from build123d import *

# Parameters (mm, degrees)
F0_W     = 90
F0_H     = 11
F0_R     = 2.15
F0_R_2   = 2.25
F1_DEPTH = 7
F2_W     = 5
F2_H     = 5
F3_DEPTH = 8
F4_R     = 5
F5_R     = 2.99999


# Not quite as in the source:
# - a fillet or chamfer is up to 0.001 mm smaller than in the source, because OpenCascade refuses the exact size


with BuildPart() as f1:
    # F0 (on Top) → F1 (new body)
    with BuildSketch(Plane.XY):
        Rectangle(F0_W, F0_H)
        with Locations((-40, 0)):
            Circle(F0_R, mode=Mode.SUBTRACT)
        Circle(F0_R_2, mode=Mode.SUBTRACT)
        with Locations((40, 0)):
            Circle(F0_R, mode=Mode.SUBTRACT)
        Circle(F0_R_2)
    extrude(amount=F1_DEPTH)

    # F2 (on face) → F3 (join)
    with BuildSketch(Plane.XY.offset(7)):
        Rectangle(F2_W, F2_H)
    extrude(amount=F3_DEPTH)

    # F4
    f4_edges = [f1.edges().sort_by_distance(p)[0] for p in [
        (45, -5.5, 3.5),
        (45, 5.5, 3.5),
        (-45, -5.5, 3.5),
        (-45, 5.5, 3.5),
    ]]
    fillet(f4_edges, radius=F4_R)

    # F5 (radius 3 in the source; OpenCascade refuses exactly that, so slightly less here)
    f5_edges = [f1.edges().sort_by_distance(p)[0] for p in [
        (0, -5.5, 7),
    ]]
    fillet(f5_edges, radius=F5_R)


solid = f1.part
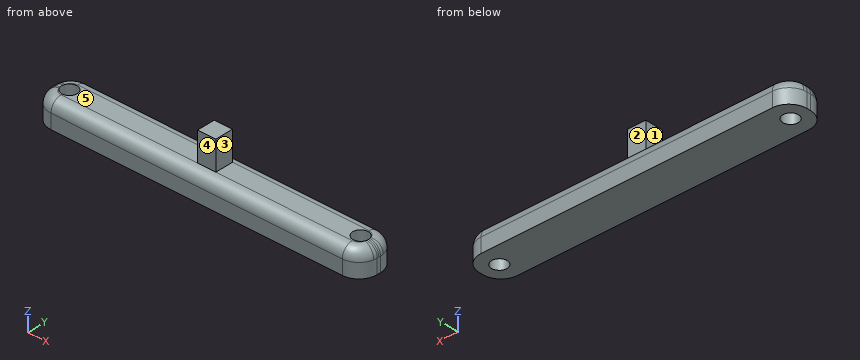
Design review of the part built by this model. Coordinates are the model's own, in mm. Face numbers are marked on the shaded views. A direction names the side the tool comes from. Coordinates: 2 decimals unless noted, no trailing zeros. Order: outer loops, then holes, each group sorted by start corner. A loop starts at its lowest first (then second) coordinate and runs counter-clockwise, first axis right, second up. Notation, with made-up numbers: (73.5, 78) -> (112.5, 78) arc R14 cw to (112.5, 95) -> close; hole circle Ø5 at (11.25, 63.25). An arc over 180 degrees is marked (long way). Use one line per item in the form item = value. Start each with the question number.
(1) For probe 1 along Y at (x, z) = (-40, 2); probe 2 along X at (y, z) = (2, 13.5); probe 3 along Z at (x, y) = (28.5, -1), list the stretches that pass through material, from the lowest coordinate up.
(2) For the marked faces 1, 2, 3, 4 and 5, list the 3-axis set-ups (+Z, -Z, +X, -X, +Y, -Y) from which the entire face can be reached by the end or side of a thin tool; tool diameter is ignored.
(3) Add section A-A on x = 22. State the section outline as (y, z) points, plus the area to 3 significant figures.
(4) Insertion check: pin 1 (1.5 mm diameter, centred on x = 0.5, z = 11, fed in from +Y); pin 2 (1.5 mm diameter, centred on y = 0.5, z = 12.5, fed in from +X); pin 3 (1.5 mm diameter, centred on x = -29.5, z = 7, fed in from +Y). Each pin has a flat end and moves straight along its axis. Give the tip position at first contact, or say it passes through.
(5) Add section B-B on z = 11.75. State the section outline as (x, y) points.
Answer block:
q1.probe_1 = -5.5 to -2.15, 2.15 to 5.5
q1.probe_2 = -2.5 to 2.5
q1.probe_3 = 0 to 7
q2.face_1 = +Z, -X, +Y, -Y
q2.face_2 = +Z, +X, -X, +Y
q2.face_3 = +Z, +X, +Y, -Y
q2.face_4 = +Z, +X, -X, -Y
q2.face_5 = +Z, -X, +Y, -Y
q3.outline = (-5.5, 0) -> (5.5, 0) -> (5.5, 4) arc R3 ccw to (2.5, 7) -> (-2.5, 7) arc R3 ccw to (-5.5, 4) -> close
q3.area = 73.1 mm²
q4.pin_1 = 2.5
q4.pin_2 = 2.5
q4.pin_3 = 4.48
q5.outline = (-2.5, -2.5) -> (2.5, -2.5) -> (2.5, 2.5) -> (-2.5, 2.5) -> close
